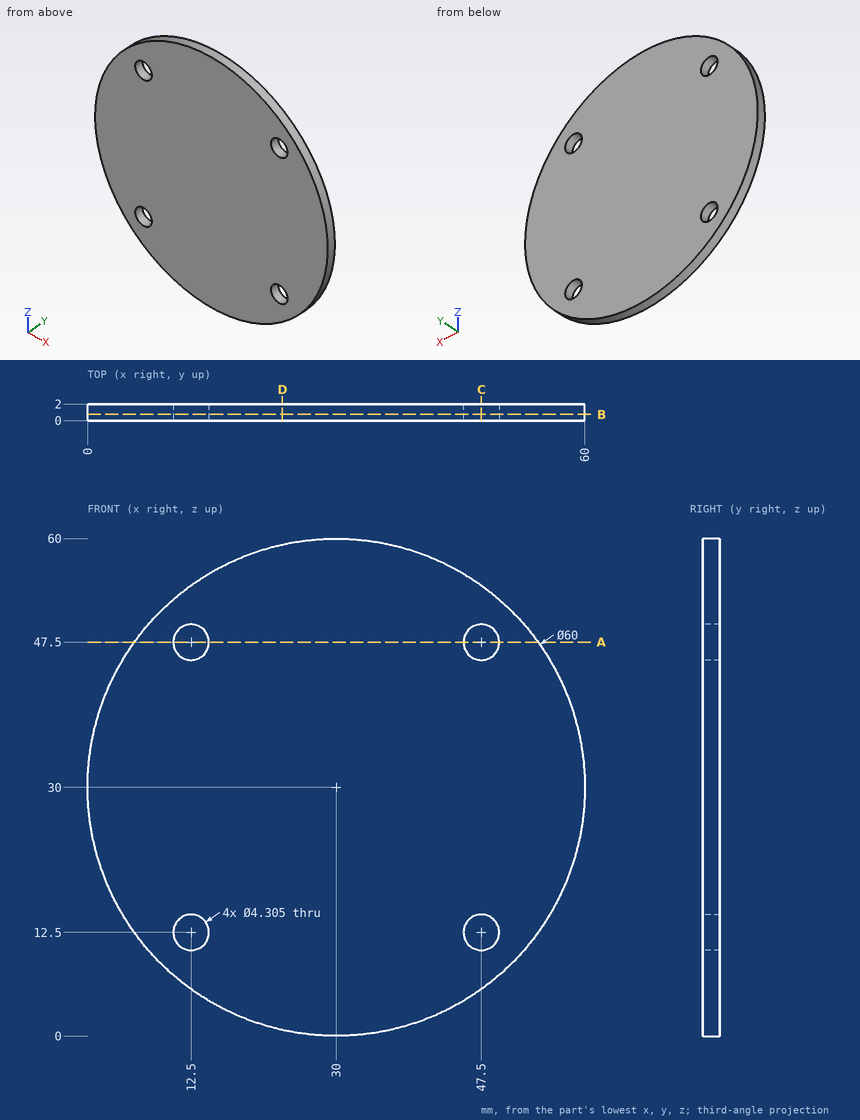
Check sheet for the drawn part. Datum: minimum x, y, z corner. Units: mm. Give positions to 0.01 mm unless a question says otherwise; leave off trailing zeros. Order: outer loops, then holes, each group sorted by start corner. A loop starts at its lowest first (then second) coordinate and runs counter-clockwise, first axis right, second up. Notation, with made-up numbers: (55.25, 54.25) -> (65.25, 54.25) arc R12 cw to (65.25, 65.25) -> close; hole circle Ø1 at (-15.5, 70.5). An arc over 180 degrees is marked (long way). One line per item, written item: value.
(1) Scan lines: line 1 along Z through (x, y) = (47.5, 1.1); line 2 along X through (y, z) = (0.4, 30); line 3 along Z through (x, y) = (20, 0.45) (1 decimal). Record each from-to range of solid material in increasing order. Write a range as [from, to].
Final values:
line 1: [5.63, 10.35], [14.65, 45.35], [49.65, 54.37]
line 2: [0, 60]
line 3: [1.7, 58.3]
(2) Sectioned sample at D-D on x = 23.5. Record the cut outline in (y, z), then the cut area to 3 significant figures.
Final values:
outline: (0, 0.71) -> (2, 0.71) -> (2, 59.29) -> (0, 59.29) -> close
area: 117 mm^2
(3) Sectioned sample at A-A on z = 47.5. Record the cut outline in (x, y).
Final values:
outline: (5.63, 0) -> (10.35, 0) -> (10.35, 2) -> (5.63, 2) -> close; (14.65, 0) -> (45.35, 0) -> (45.35, 2) -> (14.65, 2) -> close; (49.65, 0) -> (54.37, 0) -> (54.37, 2) -> (49.65, 2) -> close
(4) Sectioned sample at C-C on x = 47.5. Record the cut outline in (y, z).
Final values:
outline: (0, 5.63) -> (2, 5.63) -> (2, 10.35) -> (0, 10.35) -> close; (0, 14.65) -> (2, 14.65) -> (2, 45.35) -> (0, 45.35) -> close; (0, 49.65) -> (2, 49.65) -> (2, 54.37) -> (0, 54.37) -> close
(5) Sectioned sample at B-B on y = 0.75. Record the cut outline in (x, z) (1 decimal), then the cut area to 3 significant figures.
Final values:
outline: circle Ø60 at (30, 30); hole circle Ø4.3 at (12.5, 12.5); hole circle Ø4.3 at (12.5, 47.5); hole circle Ø4.3 at (47.5, 12.5); hole circle Ø4.3 at (47.5, 47.5)
area: 2,770 mm^2
